from build123d import *

# Parameters (mm, degrees)
BOSS_EXTRUDE1_DEPTH = 3
BOSS_EXTRUDE2_DEPTH = 2
CUT_EXTRUDE1_DEPTH  = 17.476650145
SKETCH6_R           = 3.5
SKETCH6_R_2         = 2.65
CUT_EXTRUDE3_DEPTH  = 1
BOSS_EXTRUDE4_START = 1
SKETCH7_R           = 2.65
BOSS_EXTRUDE4_DEPTH = 1
BOSS_EXTRUDE5_START = 1
SKETCH8_R           = 4.5
SKETCH8_R_2         = 3.5
BOSS_EXTRUDE5_DEPTH = 1
SKETCH9_R           = 1.25
BOSS_EXTRUDE6_DEPTH = 10.9
CHAMFER2_SIZE       = 1


with BuildPart() as part:
    # Sketch1 → Boss-Extrude1 (new body)
    with BuildSketch(Plane(origin=(0, 0, 0), x_dir=(1, 0, 0), z_dir=(0, 1, 0))):
        with BuildLine():
            Line((1, 0), (8.4, 0))
            ThreePointArc((8.4, 0), (9.107106781, 0.292893219), (9.4, 1))
            Line((9.4, 1), (9.4, 4.4))
            ThreePointArc((9.4, 4.4), (9.107106781, 5.107106781), (8.4, 5.4))
            Line((8.4, 5.4), (1, 5.4))
            ThreePointArc((1, 5.4), (0.292893219, 5.107106781), (0, 4.4))
            Line((0, 4.4), (0, 1))
            ThreePointArc((0, 1), (0.292893219, 0.292893219), (1, 0))
        make_face()
    extrude(amount=BOSS_EXTRUDE1_DEPTH)

    # Sketch2 → Boss-Extrude2 (add)
    with BuildSketch(Plane.XZ):
        with BuildLine():
            Line((1, -7.8), (8.4, -7.8))
            ThreePointArc((8.4, -7.8), (10.804163056, -6.804163056), (11.8, -4.4))
            Line((11.8, -4.4), (11.8, -1))
            ThreePointArc((11.8, -1), (10.804163056, 1.404163056), (8.4, 2.4))
            Line((8.4, 2.4), (1, 2.4))
            ThreePointArc((1, 2.4), (-1.404163056, 1.404163056), (-2.4, -1))
            Line((-2.4, -1), (-2.4, -4.4))
            ThreePointArc((-2.4, -4.4), (-1.404163056, -6.804163056), (1, -7.8))
        make_face()
    extrude(amount=BOSS_EXTRUDE2_DEPTH)

    # Sketch3 → Cut-Extrude1 (cut, through all)
    with BuildSketch(Plane.ZY.offset(2.4)):
        with BuildLine():
            Line((-5.4, -0.1), (-5.4, 0.4))
            Line((-5.4, 0.4), (-7.8, 0.4))
            Line((-7.8, 0.4), (-7.8, -0.73))
            ThreePointArc((-7.8, -0.73), (-6.63183862, -0.29371002), (-5.4, -0.1))
        make_face()
    extrude(amount=-CUT_EXTRUDE1_DEPTH, mode=Mode.SUBTRACT)

    # Sketch6 → Cut-Extrude3 (cut)
    with BuildSketch(Plane.XZ.offset(2)):
        with Locations(Location((4.7, -2.7, 0), (0, 0, 270))):
            Circle(SKETCH6_R)
        with Locations(Location((4.7, -2.7, 0), (0, 0, 270))):
            Circle(SKETCH6_R_2, mode=Mode.SUBTRACT)
    extrude(amount=-CUT_EXTRUDE3_DEPTH, mode=Mode.SUBTRACT)

    # Sketch7 → Boss-Extrude4 (add)
    with BuildSketch(Plane.XZ.offset(2).offset(BOSS_EXTRUDE4_START)):
        with Locations(Location((4.7, -2.7, 0), (0, 0, 270))):
            Circle(SKETCH7_R)
    extrude(amount=-BOSS_EXTRUDE4_DEPTH)

    # Sketch8 → Boss-Extrude5 (add)
    with BuildSketch(Plane.XZ.offset(2).offset(BOSS_EXTRUDE5_START)):
        with Locations(Location((4.7, -2.7, 0), (0, 0, 270))):
            Circle(SKETCH8_R)
        with Locations(Location((4.7, -2.7, 0), (0, 0, 270))):
            Circle(SKETCH8_R_2, mode=Mode.SUBTRACT)
    extrude(amount=-BOSS_EXTRUDE5_DEPTH)

    # Sketch9 → Boss-Extrude6 (add)
    with BuildSketch(Plane.XZ.offset(3)):
        with Locations(Location((4.7, -2.7, 0), (0, 0, 270))):
            Circle(SKETCH9_R)
    extrude(amount=BOSS_EXTRUDE6_DEPTH)

    # Chamfer2
    chamfer2_edges = [part.edges().sort_by_distance(p)[0] for p in [
        (4.7, -3, -1.45),
    ]]
    chamfer(chamfer2_edges, length=CHAMFER2_SIZE)


solid = part.part
The listing builds one solid part. Answer for the finished solid, in the listing's coordinates (mm). A direction names the side the tool comes from. Give positions to 0.01 mm unless a question says otherwise; leave off trailing zeros. Loops run counter-clockwise (first coordinate to the right, second up) from the corner with the lowest first, then second, coordinate; pieces in that order, holes last. Notation, with made-up numbers: (52.25, 31) - (78.25, 31) arc R29 cw to (78.25, 61) - close; hole circle Ø9 at (-11.5, 75). An arc over 180 degrees is marked (long way). Use one line per item in the form item = value.
1. Section D-D on y = -12 is taken. Give the vertices of the cut face in (x, z), then the cut area to 3 significant figures.
Calculated:
outline = circle Ø2.5 at (4.7, -2.7)
area = 4.91 mm^2
2. Find the intervals of material crossed by line 1 along X through (y, z) = (-2.55, -2.7); line 2 along X through (y, z) = (-1.7, -2.7); line 3 along X through (y, z) = (0.5, -2.5), in increasing order. Write a range as [from, to].
Calculated:
line_1 = [0.2, 1.2], [2.05, 7.35], [8.2, 9.2]
line_2 = [-2.4, 1.2], [2.05, 7.35], [8.2, 11.8]
line_3 = [0, 9.4]
3. Section A-A on y = -1.5 is taken. Give the vertices of the cut face in (x, z).
Calculated:
outline = (-2.4, -4.4) arc R3.4 ccw to (1, -7.8) - (8.4, -7.8) arc R3.4 ccw to (11.8, -4.4) - (11.8, -1) arc R3.4 ccw to (8.4, 2.4) - (1, 2.4) arc R3.4 ccw to (-2.4, -1) - close; circle Ø5.3 at (4.7, -2.7); hole circle Ø7 at (4.7, -2.7)
4. Section B-B on x = 4.7 is taken. Give the vertices of the cut face in (y, z), then the cut area to 3 significant figures.
Calculated:
outline = (-13.9, -3.95) - (-4, -3.95) - (-3, -4.95) - (-3, -5.35) - (-1, -5.35) - (-1, -6.2) - (-3, -6.2) - (-3, -7.2) - (-2, -7.2) - (-2, -7.8) - (-0.73, -7.8) arc R6.2 ccw to (-0.1, -5.4) - (3, -5.4) - (3, 0) - (0, 0) - (0, 2.4) - (-2, 2.4) - (-2, 1.8) - (-3, 1.8) - (-3, 0.8) - (-1, 0.8) - (-1, -0.05) - (-3, -0.05) - (-3, -0.45) - (-4, -1.45) - (-13.9, -1.45) - close
area = 69.7 mm^2
5. The mould has two halves that part along X. Classify faces 1 (the face through (0, 1, -3)), 2 (the face through (7.33, -2.01, -2.36)), 3 (the face through (5, -13.9, -3)), 4 (the face through (9.099, 1.479, -0.285)): pulls with the +X half, pulls with the -X half, needs draft (parallel to the pull), parting line crosses it, or undercut.
Calculated:
face_1 = pulls with the -X half
face_2 = undercut
face_3 = needs draft
face_4 = pulls with the +X half
6. Given pin 1 Ø4 at (x, z) = (2, -6.5) entering from -Y; pin 2 Ø1.5 at (x, y) = (3.5, 1) entering from -Z; pin 3 Ø0.9 at (x, y) = (3.5, 1.5) entering from +Z, each flat-ended and moving along its own axis, determine where each tip first touches the part or whether it passes through.
Calculated:
pin_1 = -3
pin_2 = -5.4
pin_3 = 0
7. Which of the six approach directions +Z, -Z, +X, -X, +Y, -Y give full straight-line access (tool end or side, diameter ignored) to faces 5 (the face through (0.301, 1.479, -5.115)), 6 (the face through (5, 1, 0)), 7 (the face through (-1.38, -0.99, 1.43)), 8 (the face through (2, -3, 0))?
Calculated:
face_5 = -Z, -X, +Y
face_6 = +Z, +X, -X, +Y
face_7 = +Z, -X, +Y, -Y
face_8 = -Y
8. Section C-C on z = -2.7 is taken. Give the vertices of the cut face in (x, y).
Calculated:
outline = (-2.4, -2) - (0.2, -2) - (0.2, -3) - (1.2, -3) - (1.2, -1) - (2.05, -1) - (2.05, -3) - (2.45, -3) - (3.45, -4) - (3.45, -13.9) - (5.95, -13.9) - (5.95, -4) - (6.95, -3) - (7.35, -3) - (7.35, -1) - (8.2, -1) - (8.2, -3) - (9.2, -3) - (9.2, -2) - (11.8, -2) - (11.8, 0) - (9.4, 0) - (9.4, 3) - (0, 3) - (0, 0) - (-2.4, 0) - close
